CAD build for the part. Positions are in the model's coordinates, mm. A direction names the side the tool comes from. Round coordinates to 2 decimals unless told otherwise and drop trailing zeros. Loops run counter-clockwise (first coordinate to the right, second up) from the corner with the lowest first, then second, coordinate; pieces in that order, holes last. Notation, with made-up numbers: M 9,24.25 L 55,24.25 A20 cw 55,38.25 Z; hole C 9,-37 d7. An arc over 180 degrees is marked long. One line per item, written item: value. Start each with the question number.
from build123d import *

# Parameters (mm, degrees)
SKETCH_1_W           = 122.5
SKETCH_1_H           = 120
EXTRUDE_1_DEPTH      = 3
EXTRUDE_2_DEPTH      = 61.25
EXTRUDE_2_DEPTH_BACK = 61.25
SKETCH_5_W           = 3
SKETCH_5_H           = 55
EXTRUDE_3_DEPTH      = 3
HOLE_WIZARD_M6_1_D   = 5
EXTRUDE_4_DEPTH      = 3
HOLE_WIZARD_M4_3_D   = 3.3
SKETCH_29_W          = 31
SKETCH_29_H          = 15
SKETCH_29_W_2        = 16.3
CUT_EXTRUDE_1_DEPTH  = 169.59882117


with BuildPart() as part:
    # 草图1 → 凸台-拉伸1 (new body)
    with BuildSketch(Plane(origin=(0, 0, 0), x_dir=(1, 0, 0), z_dir=(0, 1, 0))):
        Rectangle(SKETCH_1_W, SKETCH_1_H)
    extrude(amount=EXTRUDE_1_DEPTH)

    # 草图5 → 凸台-拉伸2 (add, two sides: drawn at the far end of the back side and taken through both)
    with BuildSketch(Plane(origin=(0, 0, 0), x_dir=(0, 0, -1), z_dir=(1, 0, 0)).offset(-EXTRUDE_2_DEPTH_BACK)):
        with Locations((-61.5, -24.5)):
            Rectangle(SKETCH_5_W, SKETCH_5_H)
    extrude(amount=EXTRUDE_2_DEPTH + EXTRUDE_2_DEPTH_BACK)

    # 草图23 → 凸台-拉伸3 (add)
    with BuildSketch(Plane(origin=(0, 3, 0), x_dir=(1, 0, 0), z_dir=(0, 1, 0))):
        with BuildLine():
            Line((17, 60), (33, 60))
            Line((33, 60), (33, 72))
            ThreePointArc((33, 72), (25, 80), (17, 72))
            Line((17, 72), (17, 60))
        make_face()
        with BuildLine():
            Line((-17, 60), (-17, 72))
            ThreePointArc((-17, 72), (-25, 80), (-33, 72))
            Line((-33, 72), (-33, 60))
            Line((-33, 60), (-17, 60))
        make_face()
    extrude(amount=-EXTRUDE_3_DEPTH)

    # M6 螺纹孔1 (through all)
    with Locations(Plane(origin=(0, 3, 0), x_dir=(1, 0, 0), z_dir=(0, 1, 0))):
        with Locations((-25, 72), (25, 72)):
            Hole(HOLE_WIZARD_M6_1_D / 2)

    # 草图26 → 凸台-拉伸4 (add)
    with BuildSketch(Plane.XY.offset(63)):
        with BuildLine():
            Line((-30, -52), (-20, -52))
            Line((-20, -52), (-20, -60))
            ThreePointArc((-20, -60), (-25, -65), (-30, -60))
            Line((-30, -60), (-30, -52))
        make_face()
        with BuildLine():
            Line((30, -52), (20, -52))
            Line((20, -52), (20, -60))
            ThreePointArc((20, -60), (25, -65), (30, -60))
            Line((30, -60), (30, -52))
        make_face()
    extrude(amount=-EXTRUDE_4_DEPTH)

    # M4 螺纹孔3 (through all)
    with Locations(Plane.XY.offset(63)):
        with Locations((-25, -60)):
            hole_wizard_m4_3 = Hole(HOLE_WIZARD_M4_3_D / 2)

    # 镜向8: M4 螺纹孔3 across plane
    add(hole_wizard_m4_3.mirror(Plane(origin=(0, 0, 0), x_dir=(0, 0, 1), z_dir=(1, 0, 0))), mode=Mode.SUBTRACT)

    # 草图29 → 切除-拉伸1 (cut, through all)
    with BuildSketch(Plane.XY.offset(63)):
        with Locations((4.5, -34.5)):
            Rectangle(SKETCH_29_W, SKETCH_29_H)
        with Locations((35.52, -34.5)):
            Rectangle(SKETCH_29_W_2, SKETCH_29_H)
    extrude(amount=-CUT_EXTRUDE_1_DEPTH, mode=Mode.SUBTRACT)


solid = part.part
(1) Flat gauge pins, fed straight in: P1, Ø10, axis at y = -7.5, z = -42.5, coming from the -X side; P2, Ø1.5, axis at y = -56.5, z = 61.5, coming from the -X side; P3, Ø10, axis at x = -42, z = 10.5, coming from the -Y side; P4, Ø2.5, axis at y = 1.5, z = -67.5, coming from the -X side. Where does each tip first touch, or does it go through?
(2) Slice it at C-C, the plane z = 29.5. List the corners of the cut face in (x, y).
(3) Which spindle directions (+Z, -Z, +X, -X, +Y, -Y) get a long thin tool onto all of the face, cutting with end or side? Do faces 4 (the flat face through (-1, 0, -11)), 5 (the flat face through (-61.25, 2, 20)). Say none if no direction does.
(4) Probe L1, parallel to X at y = 1.2, z = -72; L2, parallel to Y at x = 25, z = 61.5; L3, parallel to Z at x = -25, y = 0.95. List the from-to ranges inside material, lowest first.
(5) Slice it at D-D, the plane y = -44. List the corners of the cut face in (x, z), and give its area (4 significant figures).
(6) Slice it at B-B, the plane x = 1. List the corners of the cut face in (y, z), and give its area (3 significant figures).
(7) Slice it at A-A, the plane x = 25. List the corners of the cut face in (y, z).
(8) Mould opens along Z. For faces 1 (the cylindrical face through (23.69, -61, 61.48)), 2 (the cylindrical face through (-25, 2, -80)), 3 (the cylindrical face through (-24.46, 1.48, -69.56)) say: pulls with the +Z half, pulls with the -Z half, needs draft (parallel to the pull), parting line crosses it, or undercut.
Check result:
1. P1: passes through
1. P2: stops at x = -30
1. P3: stops at y = 0
1. P4: stops at x = -33
2. outline: M -61.25,0 L 61.25,0 L 61.25,3 L -61.25,3 Z
3. face 4: -Z, +X, -X, -Y
3. face 5: +Z, -Z, -X, +Y, -Y
4. L1: x = -33 to -27.5, -22.5 to -17, 17 to 22.5, 27.5 to 33
4. L2: y = -65 to -61.65, -58.35 to 3
4. L3: z = -80 to -74.5, -69.5 to 63
5. outline: M -61.25,60 L 61.25,60 L 61.25,63 L -61.25,63 Z
5. area: 367.5 mm^2
6. outline: M -52,60 L -42,60 L -42,63 L -52,63 Z; M -27,60 L 0,60 L 0,-60 L 3,-60 L 3,63 L -27,63 Z
6. area: 480 mm^2
7. outline: M -65,60 L -61.65,60 L -61.65,63 L -65,63 Z; M -58.35,60 L 0,60 L 0,-69.5 L 3,-69.5 L 3,63 L -58.35,63 Z; M 0,-80 L 3,-80 L 3,-74.5 L 0,-74.5 Z
8. face 1: needs draft
8. face 2: pulls with the -Z half
8. face 3: undercut
